The figure shows three views and two pictorial views of one solid part (mm, origin at its lowest corner). Answer the questions. A direction names the side the tool comes from. Round coordinates to 2 decimals unless told otherwise and drop trailing zeros. Write each loop counter-clockwise with the first axis right and the second up, starting at its lowest first coordinate (ties: lowest second). Pieces come first, ordered by that corner, then holes. Notation, with made-up numbers: M 68.25,17.25 L 114.25,17.25 A21 ccw 114.25,35.25 Z; hole C 9.5,29.25 d3. An arc over 180 degrees is marked long. One line per item, written item: value. Start each with the question number.
Q1. Find section C-C (x = 8.25). Write down the section's boundary in (y, z) (1 decimal), and give its area (3 significant figures).
Q2. A tool of negligible diameter and unlimited length cuts with its end or side. For the marked faces 1, 2 and 3, from which of +Z, -Z, +X, -X, +Y, -Y can it reach the whole face along a straight path? Write none if from no direction.
Q3. Consider probe 1 along Y at (x, z) = (10, 16); probe 2 along X at (y, z) = (3, 20); probe 3 along X at (y, z) = (2, 18.5). Determine where each line is inside the solid, lowest interval first.
Q4. Find section D-D (z = 16.5). Write down the section's boundary in (x, y).
Q5. Find section A-A (z = 20). Write down the section's boundary in (x, y).
Q6. The mould has two halves that part along X. Classify the marked faces 4, 5 and 6: released by +X, released by -X, zero draft, split by the parting line, or undercut.
Q7. Given pin 1 Ø4 at (y, z) = (4.5, 24.5) entering from -X; pin 2 Ø3.5 at (x, y) = (10, 3.5) entering from +Z; pin 3 Ø3 at (y, z) = (7, 18.5) entering from +X, each flat-ended and moving along its own axis, determine where each tip first touches the part or whether it passes through.
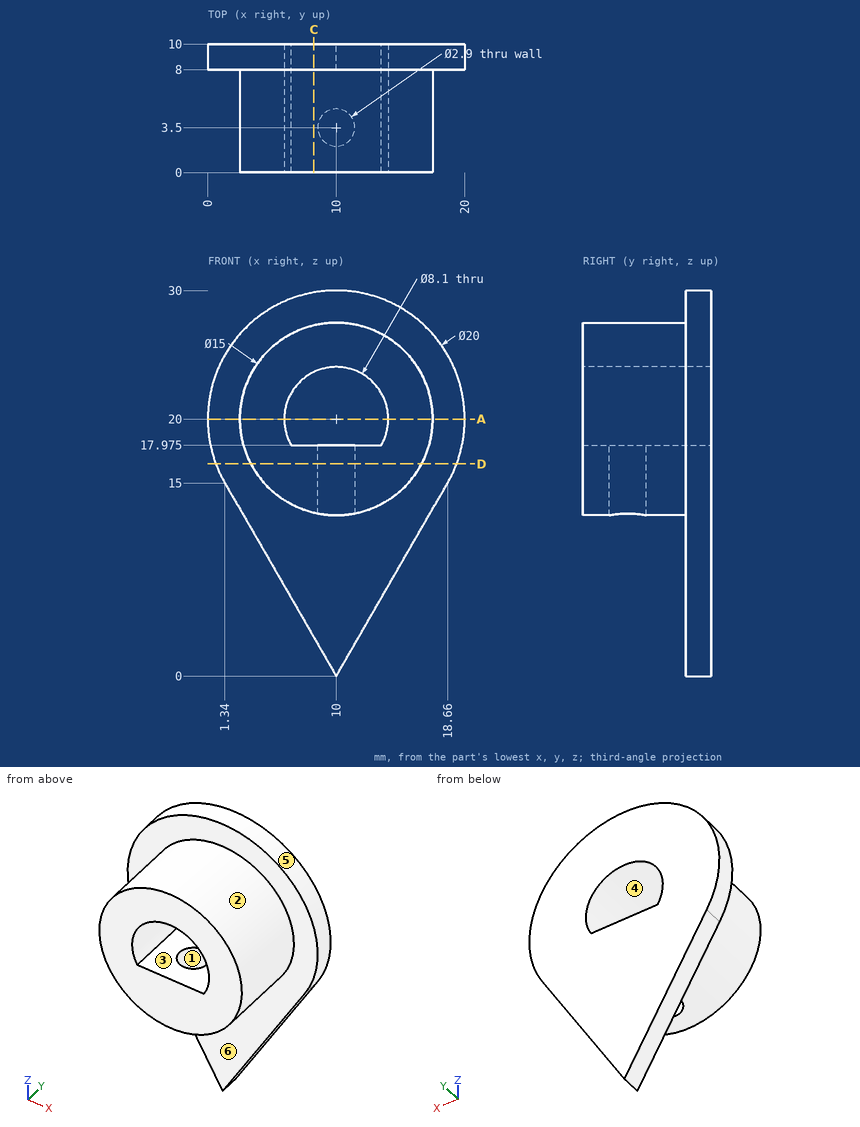
The answers:
1. outline: M 0,12.7 L 8,12.7 L 8,3 L 10,3 L 10,18 L 0,18 Z; M 0,23.7 L 10,23.7 L 10,29.8 L 8,29.8 L 8,27.3 L 0,27.3 Z
1. area: 114 mm2
2. face 1: -Z
2. face 2: -Y
2. face 3: +Y, -Y
3. probe 1: 0 to 2.05, 4.95 to 10
3. probe 2: 2.5 to 5.95, 14.05 to 17.5
3. probe 3: 2.65 to 6.24, 13.76 to 17.35
4. outline: M 0.63,8 L 3.37,8 L 3.37,0 L 16.63,0 L 16.63,8 L 19.37,8 L 19.37,10 L 0.63,10 Z; hole C 10,3.5 d2.9
5. outline: M 0,8 L 2.5,8 L 2.5,0 L 5.95,0 L 5.95,10 L 0,10 Z; M 14.05,0 L 17.5,0 L 17.5,8 L 20,8 L 20,10 L 14.05,10 Z
6. face 4: undercut
6. face 5: split by the parting line
6. face 6: zero draft
7. pin 1: x = 2.93
7. pin 2: z = 27.5
7. pin 3: x = 19.99
